```python
from build123d import *

# Parameters (mm, degrees)
BOSS_EXTRUDE1_DEPTH   = 88.3
BOSS_EXTRUDE1_2_DEPTH = 88.3
SKETCH2_W             = 103.737369208
SKETCH2_H             = 88.3
BOSS_EXTRUDE2_DEPTH   = 5
SKETCH4_W             = 25
SKETCH4_H             = 3
BOSS_EXTRUDE4_DEPTH   = 7
SKETCH6_W             = 15
SKETCH6_H             = 3
SKETCH6_H_2           = 3.987889175
CUT_EXTRUDE2_DEPTH    = 97


with BuildPart() as part:
    # Sketch1 → Boss-Extrude1 (new body)
    with BuildSketch(Plane.XY):
        Polygon((-51.868684604, 0), (-47.5, 0), (-43.131315396, 0), (-40.75, 20), (-54.25, 20), align=None)
    extrude(amount=-BOSS_EXTRUDE1_DEPTH)



with BuildPart() as body_2:
    # Sketch1 → Boss-Extrude1 2 (new body)
    with BuildSketch(Plane.XY):
        Polygon((40.75, 20), (43.131315396, 0), (47.5, 0), (51.868684604, 0), (54.25, 20), align=None)
    extrude(amount=-BOSS_EXTRUDE1_2_DEPTH)


with BuildPart() as part_1:
    add(part.part)

    add(body_2.part)  # Boss-Extrude2 merges body 2
    # Sketch2 → Boss-Extrude2 (add)
    with BuildSketch(Plane.XZ):
        with Locations((0, -44.15)):
            Rectangle(SKETCH2_W, SKETCH2_H)
    extrude(amount=BOSS_EXTRUDE2_DEPTH)

    # Sketch4 → Boss-Extrude4 (add)
    with BuildSketch(Plane.XZ.offset(5)):
        with Locations((39.368684604, -1.5)):
            Rectangle(SKETCH4_W, SKETCH4_H)
        with Locations((-11.265529701, -1.5)):
            Rectangle(SKETCH4_W, SKETCH4_H)
        with Locations((39.368684604, -85.5)):
            Rectangle(SKETCH4_W, SKETCH4_H)
        with Locations((-11.265529701, -85.5)):
            Rectangle(SKETCH4_W, SKETCH4_H)
    extrude(amount=BOSS_EXTRUDE4_DEPTH)

    # Sketch6 → Cut-Extrude2 (cut)
    with BuildSketch(Plane(origin=(0, 0, -87), x_dir=(-1, 0, 0), z_dir=(0, 0, -1))):
        with Locations((11.265529701, -6.5)):
            Rectangle(SKETCH6_W, SKETCH6_H)
        with Locations((-39.368684604, -6.993944588)):
            Rectangle(SKETCH6_W, SKETCH6_H_2)
    extrude(amount=-CUT_EXTRUDE2_DEPTH, mode=Mode.SUBTRACT)


solid = part_1.part
```
Part model, mm, in its own coordinate system. A direction names the side the tool comes from. Give positions to 0.01 mm unless a question says otherwise; leave off trailing zeros. Loops run counter-clockwise (first coordinate to the right, second up) from the corner with the lowest first, then second, coordinate; pieces in that order, holes last. Notation, with made-up numbers: M -30,21.25 L 2,21.25 A10 cw 2,36.25 Z; hole C 11,0 d1. An arc over 180 degrees is marked long. Return JSON: item names as keys, results as strings.
1) 3-axis set-ups, long thin cutter, end or side, ignore diameter. For faces 5 (the face through (-51.869, -2, -45)), 6 (the face through (31.869, -7, -2)), 7 (the face through (39.2, -9.2, -84)): which of +Z, -Z, +X, -X, +Y, -Y reach the whole face in a straight line?
Calculated:
{"face 5": "+Z, -Z, -X, -Y", "face 6": "+Z, -Z", "face 7": "+X, -X, -Y"}
2) Saw through at C-C, the plane z = -81.5. List the corners of the cut face in (x, y).
Calculated:
{"outline": "M -54.25,20 L -51.87,0 L -51.87,-5 L 51.87,-5 L 51.87,0 L 54.25,20 L 40.75,20 L 43.13,0 L -43.13,0 L -40.75,20 Z"}
3) Saw through at D-D, the plane y = 4.5. List the corners of the cut face in (x, z).
Calculated:
{"outline": "M -52.4,-88.3 L -42.6,-88.3 L -42.6,0 L -52.4,0 Z; M 42.6,-88.3 L 52.4,-88.3 L 52.4,0 L 42.6,0 Z"}
4) Flat gauge pins, fed straight in: pin 1 Ø4 at (y, z) = (-5.5, -75.5) entering from +X; pin 2 Ø8 at (x, z) = (-40.5, -17) entering from -Y; pin 3 Ø0.9 at (y, z) = (-9.5, -1) entering from -X; pin 4 Ø3.5 at (x, y) = (-15, -8) entering from +Z. Where does each tip first touch, or does it go through?
Calculated:
{"pin 1": "stops at x = 51.87", "pin 2": "stops at y = -5", "pin 3": "stops at x = -23.77", "pin 4": "stops at z = 0"}
5) Saw through at B-B, the plane y = 16.5. List the corners of the cut face in (x, z).
Calculated:
{"outline": "M -53.83,-88.3 L -41.17,-88.3 L -41.17,0 L -53.83,0 Z; M 41.17,-88.3 L 53.83,-88.3 L 53.83,0 L 41.17,0 Z"}
6) Drill centre lines: line 1 (Z direction, x = 31, y = -10); line 2 (X direction, y = 5, z = -73); line 3 (Y direction, x = 38.5, z = -27). Where is each one in solid material? Low to high.
Calculated:
{"line 1": "z = -87 to -84, -3 to 0", "line 2": "x = -52.46 to -42.54, 42.54 to 52.46", "line 3": "y = -5 to 0"}
7) Pull direction Z, two halves, no side cores. Call faces 1 (the face through (39.2, -9.2, -3)), 2 (the face through (-47, 20, -44)), 3 (the face through (-11, -9, -87)), 4 (the face through (-11, -9, -84)): released by +Z, released by -Z, zero draft, split by the parting line, or undercut.
Calculated:
{"face 1": "undercut", "face 2": "zero draft", "face 3": "released by -Z", "face 4": "undercut"}
8) Saw through at A-A, the plane y = -6.5. Count the separate pieces of the cut face and the enclosed holes in it, then the cut area to 3 significant figures.
Calculated:
{"separate pieces": "8", "enclosed holes": "0", "area": "120 mm2"}
